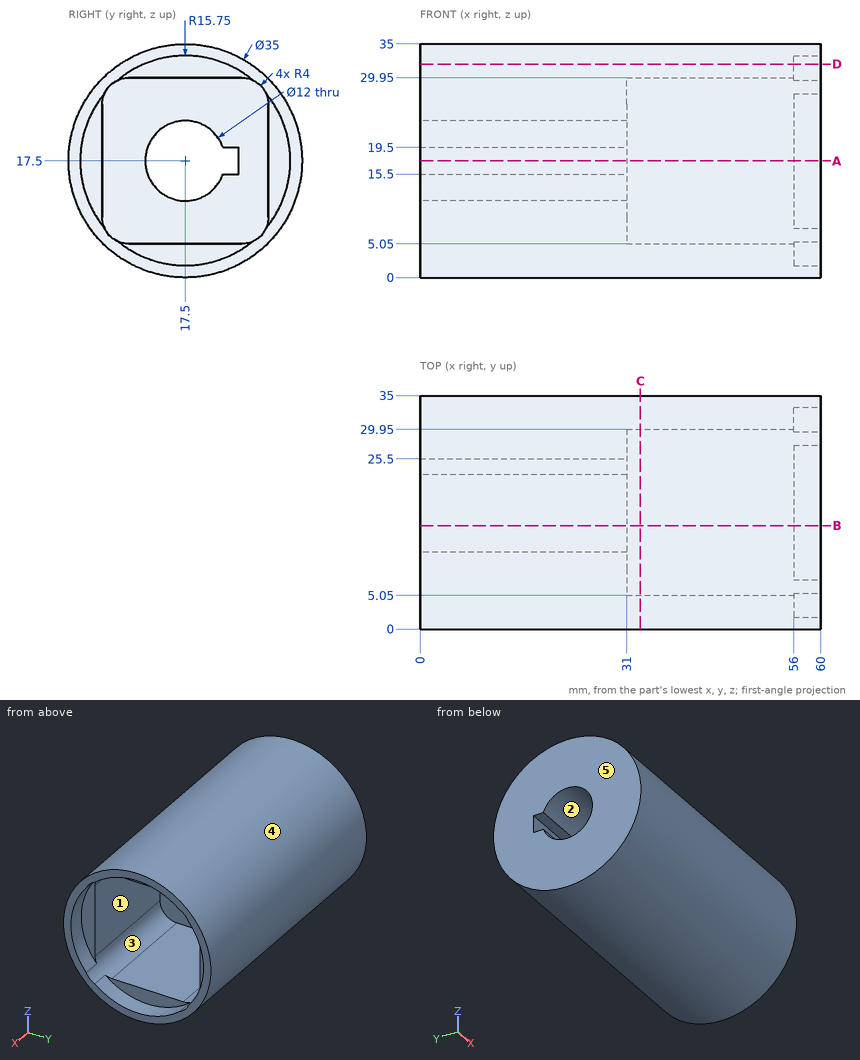
For this review, use the dimensioned drawing (mm, ordinates from the lowest corner) and the shaded views. A direction names the side the tool comes from. Coordinates: 2 decimals unless noted, no trailing zeros. Loops run counter-clockwise (first coordinate to the right, second up) from the corner with the lowest first, then second, coordinate; pieces in that order, holes last. Notation, with made-up numbers: (29.5, 51.25) - (43.5, 51.25) arc R33 cw to (43.5, 81.25) - close; hole circle Ø3 at (83, 26). An arc over 180 degrees is marked (long way). Use CSV: the item, a comma, the result in double quotes. Start each with the question number.
1) Wall thickness on L1, parallel to Y at x = 55, z = 18; L2, parallel to Y at x = 19, z = 17.5; L3, parallel to Z at x = 9, y = 25: over which ranges is each line inside the solid? List them lowest first. Write a range as from..to.
2) The part is to be moulded in two halves that separate along Y. For the marked faces 3, 4 and 5, say which applies: +Y half, -Y half, draft (parallel to the pull), parting line (faces both ways), or undercut.
3) Consider section B-B on y = 15.5. Write out the cut boundary in (x, z).
4) Consider section A-A on z = 17.5. Write out the cut boundary in (x, y), then the cut area to 4 significant figures.
5) Consider section C-C on x = 33. Write out the cut boundary in (y, z), then the cut area to 3 significant figures.
6) Tool access review of the marked faces 1 and 2: name each direction out of +Z, -Z, +X, -X, +Y, -Y from which nothing blocks a thin tool from reaching the whole face with its end or side.
7) Consider section D-D on z = 32. Write out the cut boundary in (x, y).
8) For pin 1 Ø2 at (y, z) = (14, 5) entering from +X; pin 2 Ø4 at (x, z) = (6, 5) entering from -Y; pin 3 Ø1.5 at (x, y) = (21.5, 23) entering from +Z; pin 4 Ø4 at (y, z) = (4, 21.5) entering from +X, all flat-tipped, find the tip position at first contact; note any pin that passes through.
Geometry says:
1,L1,"0.01..5.05, 29.95..34.99"
1,L2,"0..11.5, 25.5..35"
1,L3,"1.69..15.5, 19.5..33.31"
2,face 3,"undercut"
2,face 4,"parting line"
2,face 5,"draft"
3,outline,"(0, 0.11) - (60, 0.11) - (60, 1.88) - (56, 1.88) - (56, 5.05) - (31, 5.05) - (31, 11.84) - (0, 11.84) - close; (0, 23.16) - (31, 23.16) - (31, 29.95) - (56, 29.95) - (56, 33.12) - (60, 33.12) - (60, 34.89) - (0, 34.89) - close"
4,outline,"(0, 0) - (60, 0) - (60, 1.75) - (56, 1.75) - (56, 5.05) - (31, 5.05) - (31, 11.5) - (0, 11.5) - close; (0, 25.5) - (31, 25.5) - (31, 29.95) - (56, 29.95) - (56, 33.25) - (60, 33.25) - (60, 35) - (0, 35) - close"
4,area,"917.5 mm^2"
5,outline,"circle Ø35 at (17.5, 17.5); hole (5.05, 9.05) arc R4 ccw to (9.05, 5.05) - (25.95, 5.05) arc R4 ccw to (29.95, 9.05) - (29.95, 25.95) arc R4 ccw to (25.95, 29.95) - (9.05, 29.95) arc R4 ccw to (5.05, 25.95) - close"
5,area,"356 mm^2"
6,face 1,"+X"
6,face 2,"+X, -X"
7,outline,"(0, 7.7) - (60, 7.7) - (60, 11.35) - (56, 11.35) - (56, 23.65) - (60, 23.65) - (60, 27.3) - (0, 27.3) - close"
8,pin 1,"x = 56"
8,pin 2,"y = 3.5"
8,pin 3,"z = 34.34"
8,pin 4,"x = 60"
